The figure shows three views and two pictorial views of one solid part (mm, origin at its lowest corner). Answer the questions. A direction names the side the tool comes from. Round coordinates to 2 decimals unless told otherwise and drop trailing zeros. Order: outer loops, then holes, each group sorted by start corner. A loop starts at its lowest first (then second) coordinate and runs counter-clockwise, first axis right, second up. Notation, with made-up numbers: M -0.5,66 L 38.5,66 A13 ccw 38.5,82 Z; hole C 60.25,66.25 d10. An arc over 180 degrees is marked long. Return JSON: item names as keys, results as strings.
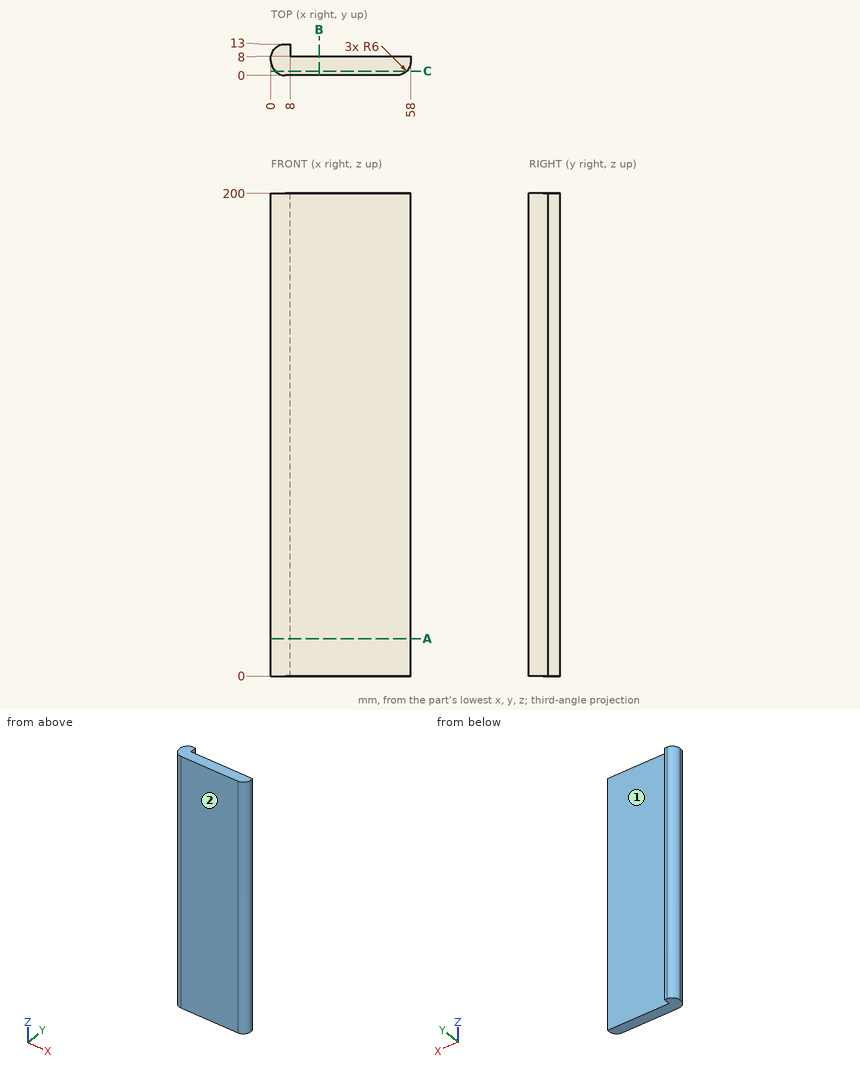
Item 1: Find section B-B (x = 20). Determine the outline of the cut face in (y, z).
Output:
{"outline": "M 0,0 L 8,0 L 8,200 L 0,200 Z"}
Item 2: Which of the six approach directions +Z, -Z, +X, -X, +Y, -Y give full straight-line access (tool end or side, diameter ignored) to the marked faces 1 and 2?
Output:
{"face 1": "+Z, -Z, +X, +Y", "face 2": "+Z, -Z, +X, -X, -Y"}
Item 3: Find section A-A (z = 15.5). Determine the outline of the cut face in (x, y).
Output:
{"outline": "M 0,6 A6 ccw 6,0 L 52,0 A6 ccw 58,6 L 58,8 L 8,8 L 8,13 L 6,13 A6 ccw 0,7 Z"}
Item 4: Consider line 1 along X through (y, z) = (7.5, 184); line 2 along Y through (x, z) = (39.5, 50); line 3 along Y through (x, z) = (5.5, 142.5). Determine where each line is inside the solid, lowest interval first. Write a range as [from, to].
Output:
{"line 1": "x = [0.02, 58]", "line 2": "y = [0, 8]", "line 3": "y = [0.02, 12.98]"}
Item 5: Each of these flat-tipped pins is pushed along its axis until it touches: pin 1 (4 mm diameter, centred on x = 21.5, z = 64.5, fed in from +Y); pin 2 (2.5 mm diameter, centred on y = 10, z = 137, fed in from +X); pin 3 (1 mm diameter, centred on y = 1.5, z = 165, fed in from +X). Where does it stop, or does it pass through?
Output:
{"pin 1": "stops at y = 8", "pin 2": "stops at x = 8", "pin 3": "stops at x = 56.47"}
Item 6: Find section C-C (y = 1.75). Determine the outline of the cut face in (x, z).
Output:
{"outline": "M 1.76,0 L 56.24,0 L 56.24,200 L 1.76,200 Z"}
